Design review of the part shown in the three views and the two pictorial views. Dimensions are in mm from the part's minimum x, y and z. Coordinates: 2 decimals unless noted, no trailing zeros. Order: outer loops, then holes, each group sorted by start corner. A loop starts at its lowest first (then second) coordinate and runs counter-clockwise, first axis right, second up. Notation, with made-up numbers: (58, 49.5) - (66, 49.5) arc R20 ccw to (66, 79.5) - close; hole circle Ø7 at (3, -37). An arc over 180 degrees is marked (long way). One line per item, written item: value. Start each with the question number.
(1) Consider section A-A on z = 0.9. Write out the cut boundary in (x, y) (1 decimal).
(2) To check wall thickness, follow line 1 along X through (y, z) = (19, 1.8) (1 decimal); line 2 along Y through (x, z) = (25, 1.7); line 3 along Y through (x, z) = (30, 3.05) (1 decimal). State the ranges of each line that lie inside material, in increasing order.
(3) Mouldability with a two-part tool opening along X and no side actions: class the marked faces 1 and 2 as released by +X, released by -X, zero draft, split by the parting line, or undercut.
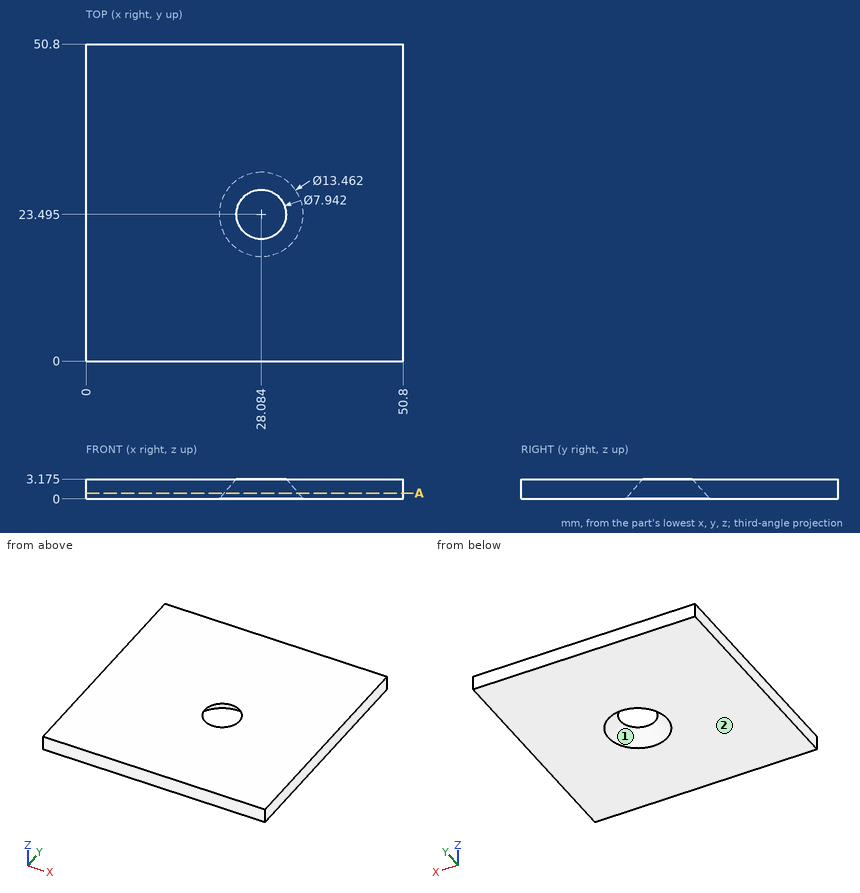
Geometry check:
1. outline: (0, 0) - (50.8, 0) - (50.8, 50.8) - (0, 50.8) - close; hole circle Ø11.9 at (28.1, 23.5)
2. line 1: x = 0 to 25.5, 30.6 to 50.8
2. line 2: y = 0 to 19.24, 27.75 to 50.8
2. line 3: y = 0 to 19.9, 27.1 to 50.8
3. face 1: undercut
3. face 2: zero draft
